Geometry check sheet. Reference: drawing and pictorial views, mm from the part's lowest x, y, z. A direction names the side the tool comes from. Round coordinates to 2 decimals unless told otherwise and drop trailing zeros. Write each loop counter-clockwise with the first axis right and the second up, starting at its lowest first coordinate (ties: lowest second). Pieces come first, ordered by that corner, then holes.
Item 1: Release check for a two-part mould opening along Z. For the marked faces 1, 2 and 3 record: pulls with the +Z half, pulls with the -Z half, needs draft (parallel to the pull), parting line crosses it, or undercut.
Item 2: Section check B-B, the plane z = 7. Record the cut outline in (x, y) (1 decimal), plus the area to 3 significant figures.
Item 3: Section check A-A, the plane x = 5.75. Record the cut outline in (y, z).
Item 4: Set-up check for the marked faces 4, 5 and 6: record each of +Z, -Z, +X, -X, +Y, -Y from which the full face is reachable in a straight line by a thin tool's end or side.
Item 5: Material ranges on line 1 along Z through (x, y) = (10, 10.4); line 2 along Z through (x, y) = (16, 11.5) (1 decimal); line 3 along Y through (x, z) = (15, 15.5), recorded low to high.
Item 6: Depth check by flat-ended pin: pin 1 (8 mm diameter, centred on x = 14.5, z = 12, fed in from +Y); pin 2 (6 mm diameter, centred on x = 8, y = 15, fed in from +Z); pin 3 (3 mm diameter, centred on x = 3.5, z = 14.5, fed in from -Y); pin 4 (6 mm diameter, centred on x = 6.5, z = 9.5, fed in from -Y). Enter the tip coordinate at first touch or a pass-through.
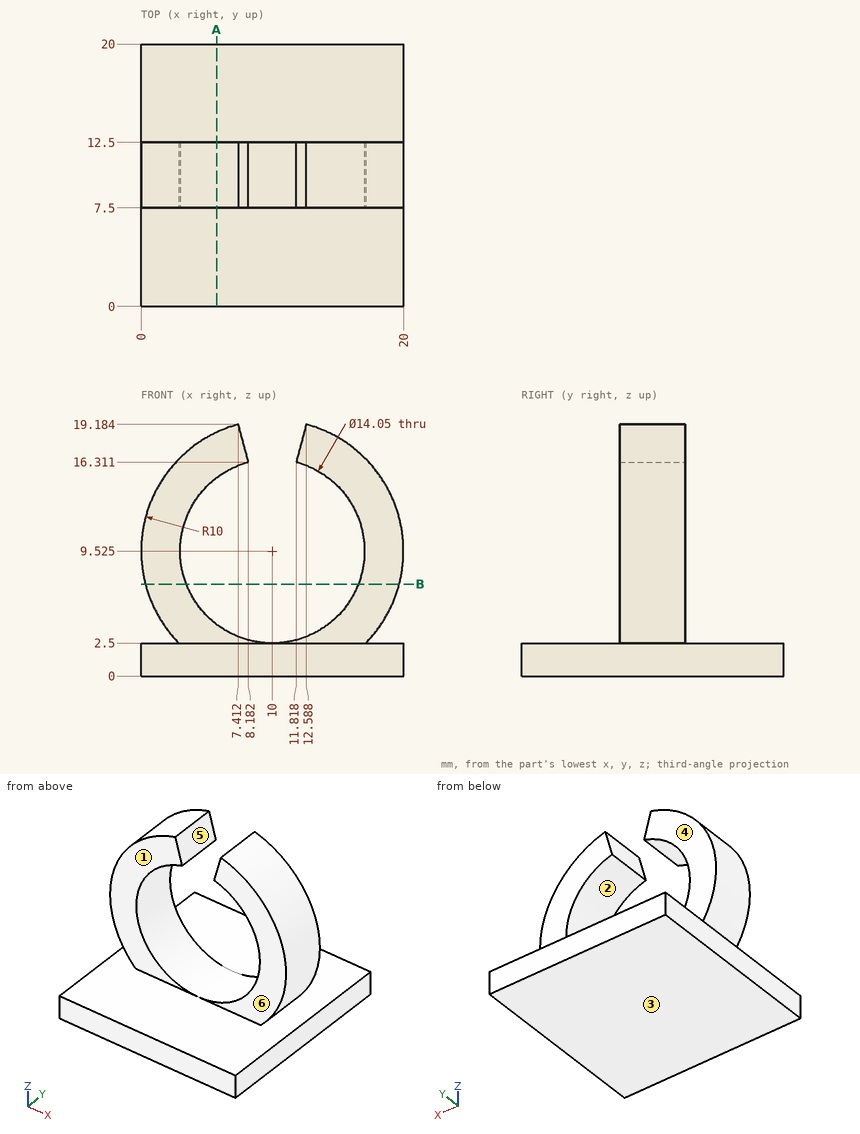
Values found:
1. face 1: needs draft
1. face 2: undercut
1. face 3: pulls with the -Z half
2. outline: (0.3, 7.5) - (3.4, 7.5) - (3.4, 12.5) - (0.3, 12.5) - close; (16.6, 7.5) - (19.7, 7.5) - (19.7, 12.5) - (16.6, 12.5) - close
2. area: 31.2 mm2
3. outline: (0, 0) - (20, 0) - (20, 2.5) - (12.5, 2.5) - (12.5, 3.93) - (7.5, 3.93) - (7.5, 2.5) - (0, 2.5) - close; (7.5, 15.12) - (12.5, 15.12) - (12.5, 18.58) - (7.5, 18.58) - close
4. face 4: +Z, +X, -X, +Y
4. face 5: +Z, +Y, -Y
4. face 6: +Z, +X, -X, -Y
5. line 1: z = 0 to 2.5
5. line 2: z = 0 to 5.9, 13.2 to 17.5
5. line 3: y = 7.5 to 12.5
6. pin 1: stops at y = 12.5
6. pin 2: stops at z = 19.18
6. pin 3: stops at y = 7.5
6. pin 4: passes through
